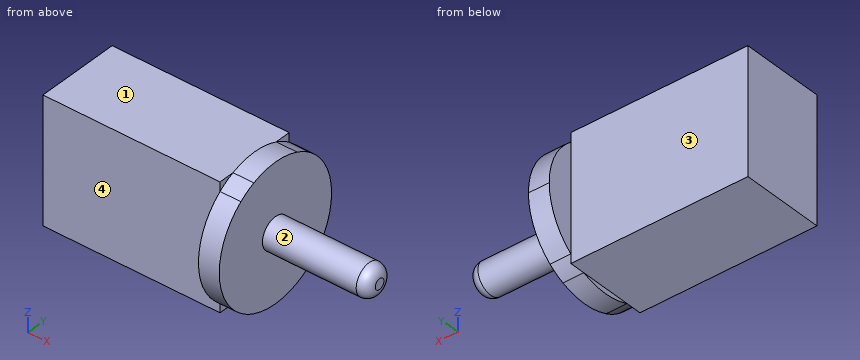
from build123d import *

# Parameters (mm, degrees)
F0_W     = 17
F0_H     = 12
F1_DEPTH = 8
F3_DEPTH = 2
F4_R     = 1.5
F5_DEPTH = 10
F6_R     = 1


with BuildPart() as f1:
    # F0 (on Front) → F1 (new body)
    with BuildSketch(Plane.XZ):
        Rectangle(F0_W, F0_H)
    extrude(amount=F1_DEPTH)

    # F2 (on face) → F3 (join)
    with BuildSketch(Plane.YZ.offset(8.5)):
        with BuildLine():
            Line((0, -5.123475383), (0, 5.123475383))
            ThreePointArc((0, 5.123475383), (-0.7205833063, 5.6120785943), (-1.5, 6))
            Line((-1.5, 6), (-6.5, 6))
            ThreePointArc((-6.5, 6), (-7.2794166937, 5.6120785943), (-8, 5.123475383))
            Line((-8, 5.123475383), (-8, -5.123475383))
            ThreePointArc((-8, -5.123475383), (-7.2794166937, -5.6120785943), (-6.5, -6))
            Line((-6.5, -6), (-1.5, -6))
            ThreePointArc((-1.5, -6), (-0.7205833063, -5.6120785943), (0, -5.123475383))
        make_face()
        with BuildLine():
            ThreePointArc((0, -5.123475383), (1.8416607228, -2.8504385627), (2.5, 0))
            ThreePointArc((2.5, 0), (1.8416607228, 2.8504385627), (0, 5.123475383))
            Line((0, 5.123475383), (0, -5.123475383))
        make_face()
        with BuildLine():
            Line((-6.5, 6), (-1.5, 6))
            ThreePointArc((-1.5, 6), (-4, 6.5), (-6.5, 6))
        make_face()
        with BuildLine():
            Line((-8, -5.123475383), (-8, 5.123475383))
            ThreePointArc((-8, 5.123475383), (-10.5, 0), (-8, -5.123475383))
        make_face()
        with BuildLine():
            ThreePointArc((-6.5, -6), (-4, -6.5), (-1.5, -6))
            Line((-1.5, -6), (-6.5, -6))
        make_face()
    extrude(amount=F3_DEPTH)

    # F4 (on face) → F5 (join)
    with BuildSketch(Plane.YZ.offset(10.5)):
        with Locations((-4, 0)):
            Circle(F4_R)
    extrude(amount=F5_DEPTH)

    # F6
    f6_edges = [f1.edges().sort_by_distance(p)[0] for p in [
        (20.5, -5.5, 0),
    ]]
    fillet(f6_edges, radius=F6_R)


solid = f1.part
Model file for the job. Use its own axes, mm. Face numbers are marked on the shaded views. A direction names the side the tool comes from. Give positions to 0.01 mm unless a question says otherwise; leave off trailing zeros. Order: outer loops, then holes, each group sorted by start corner. A loop starts at its lowest first (then second) coordinate and runs counter-clockwise, first axis right, second up. Notation, with made-up numbers: (-1, -14) - (35, -14) arc R12 ccw to (35, -7) - close; hole circle Ø6 at (81.25, 5). An arc over 180 degrees is marked (long way). Write item = value, one per line. Start each with the question number.
1. Drop flat-ended pins along their axis: P1, Ø0.7, axis at y = -1, z = 5.5, coming from the +X side; P2, Ø6, axis at x = 10.5, y = -5, coming from the -Z side; P3, Ø0.6, axis at y = -5, z = 6.5, coming from the -X side; P4, Ø2.5, axis at x = 1.5, y = -5, coming from the +Z side. Give the stop position or say it passes through.
2. Cut at C-C, the plane x = 7. List the corners of the cut face in (y, z), and give its area (3 significant figures).
3. Cut at D-D, the plane y = -8.5. List the corners of the cut face in (x, z).
4. Which spindle directions (+Z, -Z, +X, -X, +Y, -Y) get a long thin tool onto all of the face, cutting with end or side? Do the marked faces 1, 2, 3 and 4. Say none if no direction does.
5. Cut at B-B, the plane y = -6. List the corners of the cut face in (x, z).
6. Cut at A-A, the plane z = -4. List the corners of the cut face in (x, y), and give its area (3 significant figures).
7. Probe line 1 along X through (y, z) = (-7.25, 1); line 2 along X through (y, z) = (1.5, -3); line 3 along Z through (x, y) = (3.5, -0.25). List the from-to ranges inside material, lowest first.
Taken from the geometry:
q1.P1 = 10.5
q1.P2 = -6.5
q1.P3 = 8.5
q1.P4 = 6
q2.outline = (-8, -6) - (0, -6) - (0, 6) - (-8, 6) - close
q2.area = 96.0 mm²
q3.outline = (8.5, -4.69) - (10.5, -4.69) - (10.5, 4.69) - (8.5, 4.69) - close
q4.face_1 = +Z, -X, +Y, -Y
q4.face_2 = +X
q4.face_3 = +Z, -Z, -X, +Y
q4.face_4 = +Z, -Z, -X, -Y
q5.outline = (-8.5, -6) - (8.5, -6) - (8.5, -6.18) - (10.5, -6.18) - (10.5, 6.18) - (8.5, 6.18) - (8.5, 6) - (-8.5, 6) - close
q6.outline = (-8.5, -8) - (8.5, -8) - (8.5, -9.12) - (10.5, -9.12) - (10.5, 1.12) - (8.5, 1.12) - (8.5, 0) - (-8.5, 0) - close
q6.area = 156 mm²
q7.line_1 = -8.5 to 10.5
q7.line_2 = 8.5 to 10.5
q7.line_3 = -6 to 6
